Drawing for the job (mm, zero at the part's lowest x, y, z). A direction names the side the tool comes from. Round coordinates to 2 decimals unless told otherwise and drop trailing zeros. Order: outer loops, then holes, each group sorted by start corner. A loop starts at its lowest first (then second) coordinate and runs counter-clockwise, first axis right, second up. Notation, with made-up numbers: (27, 8.5) - (60, 8.5) arc R32 ccw to (60, 36.5) - close; hole circle Ø11 at (34, 7.25). An arc over 180 degrees is marked (long way). Answer as a JSON object with one key per item and string values.
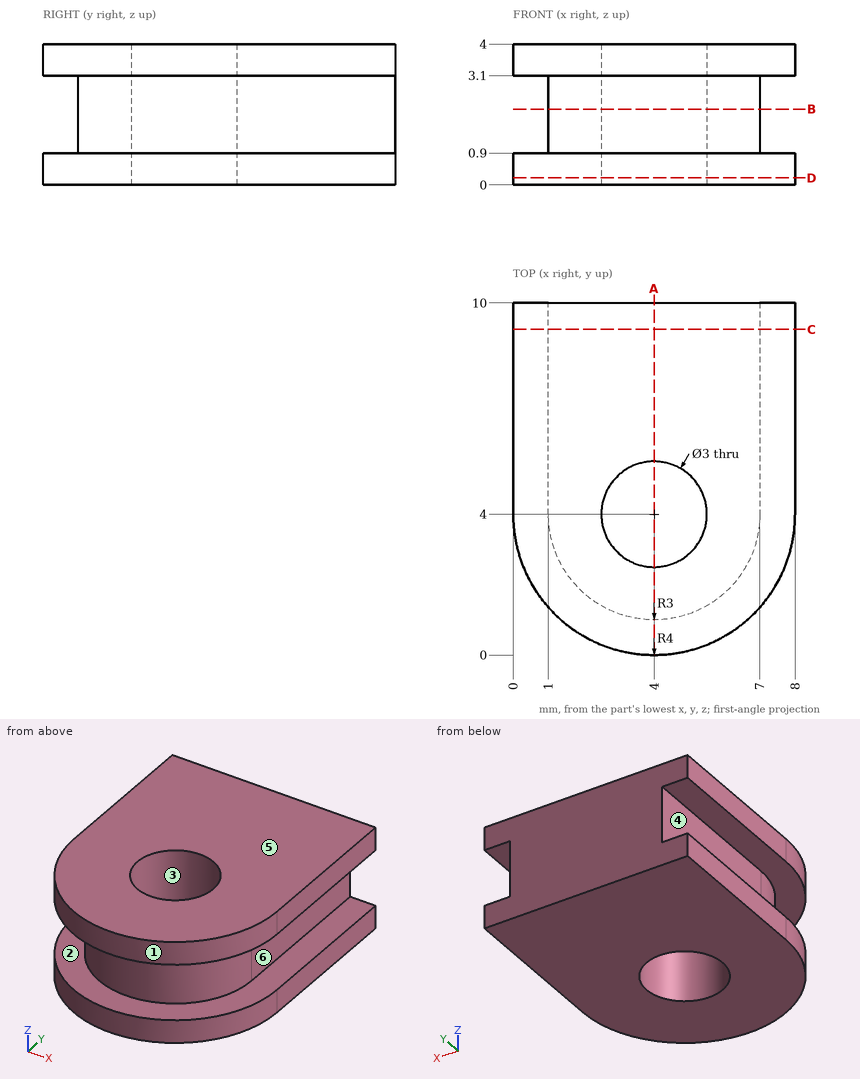
Item 1: Tool access for the marked faces 1 and 2: list every direction of +Z, -Z, +X, -X, +Y, -Y with a clear straight run to the whole face (end or side of a thin tool).
Taken from the geometry:
{"face 1": "+Z, -Z, -Y", "face 2": "-Y"}
Item 2: Cut at A-A (x = 4). Write the cut outline in (y, z), plus the area to 3 significant figures.
Taken from the geometry:
{"outline": "(0, 0) - (2.5, 0) - (2.5, 4) - (0, 4) - (0, 3.1) - (1, 3.1) - (1, 0.9) - (0, 0.9) - close; (5.5, 0) - (10, 0) - (10, 4) - (5.5, 4) - close", "area": "25.8 mm2"}
Item 3: Cut at C-C (y = 9.25). Write the cut outline in (x, z), plus the area to 3 significant figures.
Taken from the geometry:
{"outline": "(0, 0) - (8, 0) - (8, 0.9) - (7, 0.9) - (7, 3.1) - (8, 3.1) - (8, 4) - (0, 4) - (0, 3.1) - (1, 3.1) - (1, 0.9) - (0, 0.9) - close", "area": "27.6 mm2"}
Item 4: Drop flat-ended pins along their axis: P1, Ø2.5, axis at x = 4, y = 3, coming from the -Z side; P2, Ø0.7, axis at y = 7, z = 2, coming from the +X side; P3, Ø0.7, axis at y = 7.5, z = 2.5, coming from the -X side; P4, Ø1.8, axis at x = 4, y = 4, coming from the -Z side. Give the stop position or say it passes through.
Taken from the geometry:
{"P1": "z = 0", "P2": "x = 7", "P3": "x = 1", "P4": "through"}
Item 5: Probe L1, parallel to Z at x = 2.5, y = 0.5; L2, parallel to Y at x = 4, z = 1.4; L3, parallel to Y at x = 4, z = 3.55. List the from-to ranges inside material, lowest first. Write a range as from..to.
Taken from the geometry:
{"L1": "0..0.9, 3.1..4", "L2": "1..2.5, 5.5..10", "L3": "0..2.5, 5.5..10"}
Item 6: Cut at D-D (z = 0.2). Write the cut outline in (x, y).
Taken from the geometry:
{"outline": "(0, 4) arc R4 ccw to (8, 4) - (8, 10) - (0, 10) - close; hole circle Ø3 at (4, 4)"}
Item 7: Two-plate mould, pull along Z, no slides. Class the marked faces 3, 4, 5 and 6: pulls with the +Z half, pulls with the -Z half, needs draft (parallel to the pull), parting line crosses it, or undercut.
Taken from the geometry:
{"face 3": "needs draft", "face 4": "undercut", "face 5": "pulls with the +Z half", "face 6": "undercut"}
Item 8: Cut at B-B (z = 2.15). Write the cut outline in (x, y), plus the area to 3 significant figures.
Taken from the geometry:
{"outline": "(1, 4) arc R3 ccw to (7, 4) - (7, 10) - (1, 10) - close; hole circle Ø3 at (4, 4)", "area": "43.1 mm2"}
